from build123d import *

# Parameters (mm, degrees)
F0_W     = 40
F0_H     = 50
F1_DEPTH = 20
F2_DEPTH = 30
F4_DEPTH = 40
F5_DEPTH = 40


with BuildPart() as f1:
    # F0 (on Front) → F1 (new body)
    with BuildSketch(Plane.XZ):
        with BuildLine():
            ThreePointArc((0, 50), (-25, 25), (0, 0))
            Line((0, 0), (0, 12.5))
            ThreePointArc((0, 12.5), (-12.5, 25), (0, 37.5))
            Line((0, 37.5), (0, 50))
        make_face()
        with BuildLine():
            Line((0, 12.5), (0, 0))
            Line((0, 0), (20, 0))
            Line((20, 0), (20, 50))
            Line((20, 50), (0, 50))
            Line((0, 50), (0, 37.5))
            ThreePointArc((0, 37.5), (8.8388347648, 33.8388347648), (12.5, 25))
            ThreePointArc((12.5, 25), (8.8388347648, 16.1611652352), (0, 12.5))
        make_face()
        with Locations((40, 25)):
            Rectangle(F0_W, F0_H)
        with BuildLine():
            Line((60, 50), (60, 0))
            Line((60, 0), (80, 0))
            Line((80, 0), (80, 12.5))
            ThreePointArc((80, 12.5), (67.5, 25), (80, 37.5))
            Line((80, 37.5), (80, 50))
            Line((80, 50), (60, 50))
        make_face()
        with BuildLine():
            Line((80, 12.5), (80, 0))
            ThreePointArc((80, 0), (105, 25), (80, 50))
            Line((80, 50), (80, 37.5))
            ThreePointArc((80, 37.5), (88.8388347648, 33.8388347648), (92.5, 25))
            ThreePointArc((92.5, 25), (88.8388347648, 16.1611652352), (80, 12.5))
        make_face()
    extrude(amount=-F1_DEPTH)

    # F0 (on Front) → F2 (join)
    with BuildSketch(Plane.XZ):
        with Locations((40, 25)):
            Rectangle(F0_W, F0_H)
    extrude(amount=F2_DEPTH)

    # F3 (on face) → F4 (join)
    with BuildSketch(Plane.YZ.offset(60)):
        with BuildLine():
            Line((-30, 37.5), (-30, 50))
            ThreePointArc((-30, 50), (-55, 25), (-30, 0))
            Line((-30, 0), (-30, 12.5))
            ThreePointArc((-30, 12.5), (-42.5, 25), (-30, 37.5))
        make_face()
    extrude(amount=-F4_DEPTH)

    # F3 (on face) → F5 (cut)
    with BuildSketch(Plane.YZ.offset(60)):
        with BuildLine():
            ThreePointArc((-17.5, 25), (-21.1611652352, 33.8388347648), (-30, 37.5))
            Line((-30, 37.5), (-30, 12.5))
            ThreePointArc((-30, 12.5), (-21.1611652352, 16.1611652352), (-17.5, 25))
        make_face()
    extrude(amount=-F5_DEPTH, mode=Mode.SUBTRACT)


solid = f1.part
Read the model definition and answer for the solid it produces. Units are mm, in the model's axes. A direction names the side the tool comes from. Round coordinates to 2 decimals unless told otherwise and drop trailing zeros. Order: outer loops, then holes, each group sorted by start corner. A loop starts at its lowest first (then second) coordinate and runs counter-clockwise, first axis right, second up. Notation, with made-up numbers: (75, 17.25) - (117, 17.25) arc R18 cw to (117, 48.25) - close; hole circle Ø1 at (11.5, -38). An arc over 180 degrees is marked (long way). Use one line per item in the form item = value. Start each with the question number.
(1) For faces 1 (the face through (87, 0, 14)), 2 (the face through (39, 0, 0)), 3 (the face through (20, -16, 25)), determine the directions among +Z, -Z, +X, -X, +Y, -Y from which every point of the face is accessible in a straight line to the end or side of a thin tool.
(2) The part is cut by section D-D (z = 42). Give the vertices of the cut face in (x, y), then the cut area to 3 significant figures.
(3) Find the intervals of material crossed by line 1 along X through (y, z) = (1, 35); line 2 along X through (y, z) = (12.5, 36.5); line 3 along Y through (x, z) = (-2, 5.5), in increasing order. Write a range as from..to.
(4) The part is cut by section B-B (z = 16.5). Give the vertices of the cut face in (x, y).
(5) The part is cut by section C-C (x = -9). Give the vertices of the cut face in (y, z), then the cut area to 3 significant figures.
(6) The part is cut by section A-A (y = -22.5). Give the vertices of the cut face in (x, z).
(7) Flat-ended cylindrical pins translate along their axes: pin 1 Ø12 at (x, z) = (42, 41.5) entering from -Y; pin 2 Ø25 at (y, z) = (-28.5, 16) entering from -X; pin 3 Ø22.5 at (x, z) = (72, 30.5) entering from -Y. Find the tip coordinate at first contact, or state that the pin passes through.
Checked values:
q1.face_1 = +Z, -Z, +X, -Y
q1.face_2 = -Z, +X, -X, +Y, -Y
q1.face_3 = +Z, -Z, -X, -Y
q2.outline = (-18.33, 0) - (20, 0) - (20, -48.33) - (60, -48.33) - (60, 0) - (98.33, 0) - (98.33, 20) - (-18.33, 20) - close
q2.area = 4,270 mm^2
q3.line_1 = -22.91..-7.5, 7.5..72.5, 87.5..102.91
q3.line_2 = -22.2..-4.9, 4.9..75.1, 84.9..102.2
q3.line_3 = 0..20
q4.outline = (-23.51, 0) - (-9.17, 0) - (-9.17, 20) - (-23.51, 20) - close; (9.17, 0) - (20, 0) - (20, -20.83) - (60, -20.83) - (60, 0) - (70.83, 0) - (70.83, 20) - (9.17, 20) - close; (20, -53.51) - (60, -53.51) - (60, -39.17) - (20, -39.17) - close; (89.17, 0) - (103.51, 0) - (103.51, 20) - (89.17, 20) - close
q5.outline = (0, 1.68) - (20, 1.68) - (20, 16.33) - (0, 16.33) - close; (0, 33.67) - (20, 33.67) - (20, 48.32) - (0, 48.32) - close
q5.area = 586 mm^2
q6.outline = (20, 0) - (60, 0) - (60, 15) - (20, 15) - close; (20, 35) - (60, 35) - (60, 50) - (20, 50) - close
q7.pin_1 = -52.69
q7.pin_2 = 20
q7.pin_3 = 0
